```python
from build123d import *

# Parameters (mm, degrees)
EXTRUDE_1_DEPTH     = 3
SKETCH_2_R          = 1.6
CUT_EXTRUDE_1_DEPTH = 3
CUT_EXTRUDE_2_DEPTH = 81.678373806


with BuildPart() as part:
    # 草图1 → 凸台-拉伸1 (new body)
    with BuildSketch(Plane.XY):
        Polygon((-20, 0), (-30, 0), (-30, 40), (70, 40), (70, 0), (60, 0), (40, -20), (40, -30), (0, -30), (0, -20), align=None)
    extrude(amount=EXTRUDE_1_DEPTH)

    # 草图2 → 切除-拉伸1 (cut)
    with BuildSketch(Plane.XY.offset(3)):
        with Locations((10, -7)):
            Circle(SKETCH_2_R)
        with Locations((30, -7)):
            Circle(SKETCH_2_R)
        with Locations((10, -22)):
            Circle(SKETCH_2_R)
        with Locations((30, -22)):
            Circle(SKETCH_2_R)
        with Locations((-20, 10)):
            Circle(SKETCH_2_R)
        with Locations((-20, 32)):
            Circle(SKETCH_2_R)
        with Locations((0, 10)):
            Circle(SKETCH_2_R)
        with Locations((40, 10)):
            Circle(SKETCH_2_R)
        with Locations((60, 10)):
            Circle(SKETCH_2_R)
        with Locations((60, 32)):
            Circle(SKETCH_2_R)
        with Locations((40, 32)):
            Circle(SKETCH_2_R)
        with Locations((0, 32)):
            Circle(SKETCH_2_R)
    extrude(amount=-CUT_EXTRUDE_1_DEPTH, mode=Mode.SUBTRACT)

    # 草图3 → 切除-拉伸2 (cut, through all)
    with BuildSketch(Plane.XY.offset(3)):
        with BuildLine():
            Line((30, 24), (30, 4))
            ThreePointArc((30, 4), (20, -6), (10, 4))
            Line((10, 4), (10, 24))
            ThreePointArc((10, 24), (20, 34), (30, 24))
        make_face()
    extrude(amount=-CUT_EXTRUDE_2_DEPTH, mode=Mode.SUBTRACT)


solid = part.part
```
The model under review builds one solid part; all positions refer to its coordinate system, in mm. A direction names the side the tool comes from. Round coordinates to 2 decimals unless told otherwise and drop trailing zeros. Loops run counter-clockwise (first coordinate to the right, second up) from the corner with the lowest first, then second, coordinate; pieces in that order, holes last. Notation, with made-up numbers: (87, 14) -> (91, 14) arc R28 cw to (91, 45) -> close; hole circle Ø5 at (82, 80.25). An arc over 180 degrees is marked (long way). Answer in a Markdown table with one row per item.
1) Draft analysis for pull direction Y (two halves, no side actions). For faces 4 (the flat face through (10, 14, 2)), 5 (the flat face through (50, -10, 1)), 6 (the flat face through (9.6, 13.3, 3)), 7 (the flat face through (19, 40, 1)), state which applies: pulls with the +Y half, pulls with the -Y half, needs draft (parallel to the pull), parting line crosses it, or undercut.
Taken from the geometry:
| item | result |
|---|---|
| face 4 | undercut |
| face 5 | pulls with the -Y half |
| face 6 | needs draft |
| face 7 | pulls with the +Y half |
2) Consider section C-C, the plane z = 0.8. Count the separate pieces of the cut face and the enclosed holes in it, plus the area to 3 significant figures.
Taken from the geometry:
| item | result |
|---|---|
| separate pieces | 1 |
| enclosed holes | 13 |
| area | 4,790 mm² |
3) For pin 1 Ø1.5 at (x, z) = (64.5, 1) entering from -Y, flat-tipped, find the tip position at first contact; note if it passes through.
Taken from the geometry:
| item | result |
|---|---|
| pin 1 | stops at y = 0 |
4) Wall thickness on line 1 along Y through (x, z) = (60, 1.9); line 2 along Y through (x, z) = (14.5, 0.25); line 3 along X through (y, z) = (31.5, 1.4): over which ranges is each line inside the solid? List them lowest first.
Taken from the geometry:
| item | result |
|---|---|
| line 1 | y = 0 to 8.4, 11.6 to 30.4, 33.6 to 40 |
| line 2 | y = -30 to -4.35, 32.35 to 40 |
| line 3 | x = -30 to -21.52, -18.48 to -1.52, 1.52 to 13.39, 26.61 to 38.48, 41.52 to 58.48, 61.52 to 70 |
5) Consider section A-A, the plane y = 10. Write out the cut boundary in (x, z).
Taken from the geometry:
| item | result |
|---|---|
| outline | (-30, 0) -> (-21.6, 0) -> (-21.6, 3) -> (-30, 3) -> close; (-18.4, 0) -> (-1.6, 0) -> (-1.6, 3) -> (-18.4, 3) -> close; (1.6, 0) -> (10, 0) -> (10, 3) -> (1.6, 3) -> close; (30, 0) -> (38.4, 0) -> (38.4, 3) -> (30, 3) -> close; (41.6, 0) -> (58.4, 0) -> (58.4, 3) -> (41.6, 3) -> close; (61.6, 0) -> (70, 0) -> (70, 3) -> (61.6, 3) -> close |
6) Consider section B-B, the plane x = 20. Write out the cut boundary in (y, z), plus the area to 3 significant figures.
Taken from the geometry:
| item | result |
|---|---|
| outline | (-30, 0) -> (-6, 0) -> (-6, 3) -> (-30, 3) -> close; (34, 0) -> (40, 0) -> (40, 3) -> (34, 3) -> close |
| area | 90.0 mm² |
7) Consider section D-D, the plane y = -3.5. Write out the cut boundary in (x, z), plus the area to 3 significant figures.
Taken from the geometry:
| item | result |
|---|---|
| outline | (-16.5, 0) -> (13.39, 0) -> (13.39, 3) -> (-16.5, 3) -> close; (26.61, 0) -> (56.5, 0) -> (56.5, 3) -> (26.61, 3) -> close |
| area | 179 mm² |
8) Tool access review of faces 1 (the cylindrical face through (20, 34, 2)), 2 (the flat face through (-10, -10, 1)), 3 (the flat face through (65, 0, 1)): name each direction out of +Z, -Z, +X, -X, +Y, -Y from which nothing blocks a thin tool from reaching the whole face with its end or side.
Taken from the geometry:
| item | result |
|---|---|
| face 1 | +Z, -Z |
| face 2 | +Z, -Z, -X, -Y |
| face 3 | +Z, -Z, +X, -Y |
